CAD build for the part. Positions are in the model's coordinates, mm. Face numbers are marked on the shaded views. A direction names the side the tool comes from. Round coordinates to 2 decimals unless told otherwise and drop trailing zeros. Order: outer loops, then holes, each group sorted by start corner. A loop starts at its lowest first (then second) coordinate and runs counter-clockwise, first axis right, second up. Notation, with made-up numbers: (82.25, 70) -> (104.25, 70) arc R22 ccw to (104.25, 91) -> close; hole circle Ø2 at (16.5, 14). An arc over 180 degrees is marked (long way). Return JSON: item names as keys, results as strings. Group by question number.
Q1. Mould opens along Z. For the marked faces 4, 5 and 6 say: +Z half, -Z half, draft (parallel to the pull), parting line (faces both ways), or undercut.
Q2. Probe line 1 along Y through (x, z) = (-13, 0); line 2 along Y through (x, z) = (18.5, 0); line 3 along Z through (x, y) = (-20, -7). List the from-to ranges inside material, lowest first.
Q3. Cut at C-C (x = -0.5). Write the cut outline in (y, z), then the cut area to 3 significant figures.
Q4. Flat gauge pins, fed straight in: pin 1 (3 mm diameter, centred on x = 19.5, y = 50.5, fed in from +Z); pin 2 (2 mm diameter, centred on y = 36, z = -29, fed in from +X); pin 3 (8 mm diameter, centred on x = -8.5, z = 9, fed in from -Y). Where does each tip first touch, or does it go through?
Q5. Cut at B-B (z = 0). Count the separate pieces of the cut face and the enclosed holes in it, then the cut area to 3 significant figures.
Q6. Cut at A-A (x = -23). Write the cut outline in (y, z).
Q7. Which spindle directions (+Z, -Z, +X, -X, +Y, -Y) get a long thin tool onto all of the face, cutting with end or side? Do the marked faces 1, 2 and 3. Say none if no direction does.
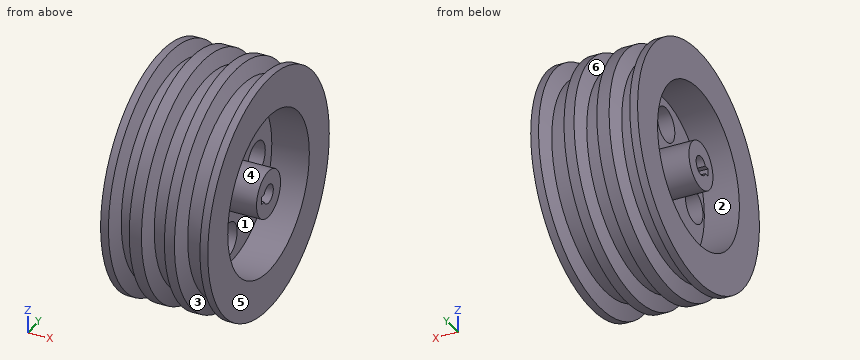
from build123d import *

# Parameters (mm, degrees)
SKETCH2_R          = 11
CUT_EXTRUDE1_DEPTH = 120.475538825
SKETCH3_W          = 5
SKETCH3_H          = 6
CUT_EXTRUDE2_DEPTH = 131.607826632


with BuildPart() as part:
    # Sketch1 → Revolve3 (revolve)
    with BuildSketch(Plane.XY):
        Polygon((35, 79.435897436), (35, 54.435897436), (11, 54.435897436), (11, 18.333333333), (35, 18.333333333), (35, 9.307692308), (-35, 9.307692308), (-35, 18.333333333), (-11, 18.333333333), (-11, 54.605542618), (-33.423992019, 54.605542618), (-33.423992019, 79.605542618), (-28.423992019, 79.605542618), (-25.019939293, 70.252984619), (-18.554189686, 70.252984619), (-15.177301066, 79.530909851), (-7.364883216, 79.530909851), (-3.96083049, 70.178351852), (3.910516857, 70.178351852), (7.287405478, 79.456277085), (13.694225587, 79.456277085), (17.226586544, 69.751195119), (26.475056629, 69.751195119), (30, 79.435897436), align=None)
    revolve(axis=Axis((74.179487179, 3.307692308, 0), (-1, 0, 0)))

    # Sketch2 → Cut-Extrude1 (cut, through all)
    with BuildSketch(Plane(origin=(11, 0, 0), x_dir=(0, 0, -1), z_dir=(1, 0, 0))):
        with Locations(Location((0, 35.256915145, 0), (0, 0, 90))):
            Circle(SKETCH2_R)
        with Locations(Location((35.256915145, 0, 0), (0, 0, 90))):
            Circle(SKETCH2_R)
        with Locations(Location((0, -35.256915145, 0), (0, 0, 90))):
            Circle(SKETCH2_R)
        with Locations(Location((-35.256915145, 0, 0), (0, 0, 90))):
            Circle(SKETCH2_R)
    extrude(amount=-CUT_EXTRUDE1_DEPTH, mode=Mode.SUBTRACT)

    # Sketch3 → Cut-Extrude2 (cut, through all)
    with BuildSketch(Plane.ZY.offset(35)):
        with Locations((0, -2.692307692)):
            Rectangle(SKETCH3_W, SKETCH3_H)
    extrude(amount=-CUT_EXTRUDE2_DEPTH, mode=Mode.SUBTRACT)


solid = part.part
Solution:
{
 "1": {"face 4": "undercut", "face 5": "draft", "face 6": "parting line"},
 "2": {"line 1": "y = -72.92 to -47.99, -11.72 to -5.69, 9.31 to 18.33, 54.61 to 79.53", "line 2": "y = -63.14 to -47.82, -11.72 to -5.69, 9.31 to 18.33, 54.44 to 69.75", "line 3": "z = -66.15 to -50.25, -10.93 to 10.93, 50.25 to 66.15"},
 "3": {"outline": "circle Ø133.74 at (3.31, 0); hole circle Ø22 at (-35.26, 0); hole circle Ø22 at (0, -35.26); hole circle Ø22 at (0, 35.26); hole (-5.69, -2.5) -> (-2.15, -2.5) arc R6 ccw (long way) to (-2.15, 2.5) -> (-5.69, 2.5) -> close; hole circle Ø22 at (35.26, 0)", "area": "12,400 mm²"},
 "4": {"pin 1": "stops at z = 48.24", "pin 2": "stops at x = 11", "pin 3": "stops at y = -72.75"},
 "5": {"separate pieces": "4", "enclosed holes": "0", "area": "4,460 mm²"},
 "6": {"outline": "circle Ø133.89 at (3.31, 0); circle Ø30.05 at (3.31, 0); hole circle Ø102.6 at (3.31, 0); hole (-5.69, -2.5) -> (-2.15, -2.5) arc R6 ccw (long way) to (-2.15, 2.5) -> (-5.69, 2.5) -> close"},
 "7": {"face 1": "+X", "face 2": "-X", "face 3": "none"}
}
